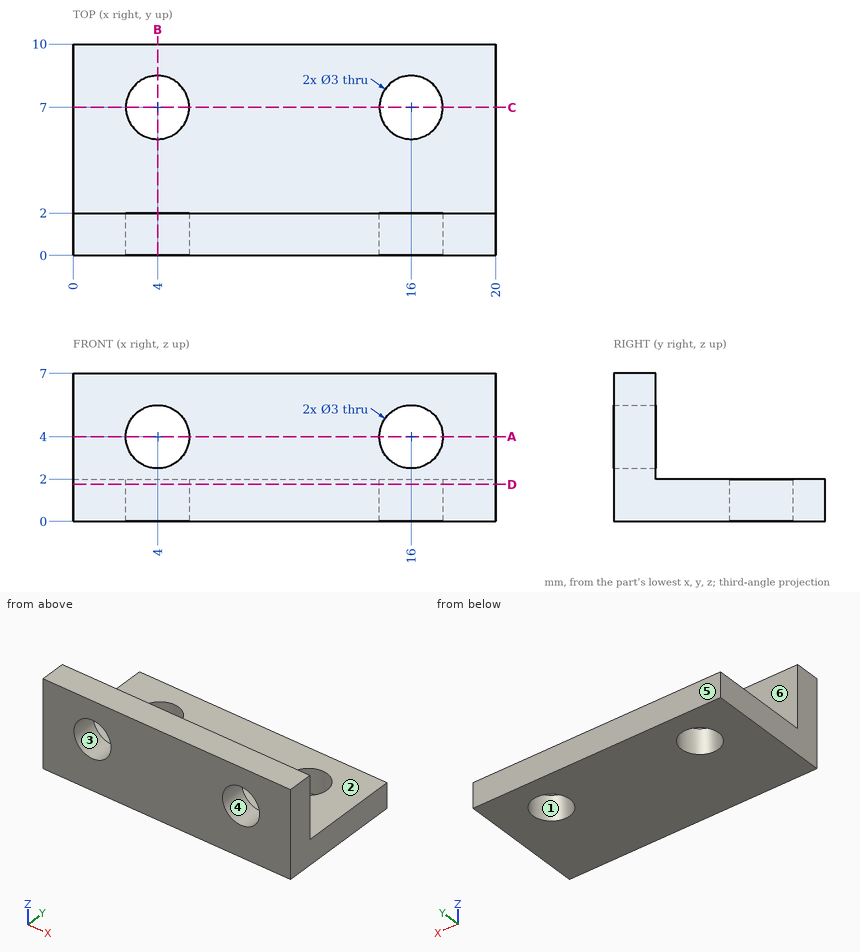
Part print with two shaded views. Sizes in mm from the minimum x, y, z corner. A direction names the side the tool comes from. Round coordinates to 2 decimals unless told otherwise and drop trailing zeros. Order: outer loops, then holes, each group sorted by start corner. A loop starts at its lowest first (then second) coordinate and runs counter-clockwise, first axis right, second up.
(1) Band-saw the part on B-B (x = 4). List the corners of the cut face in (y, z), then the cut area to 3 significant figures.
(2) Pin check, flat tips, straight feed: pin 1 (1 mm diameter, centred on x = 17.5, z = 5, fed in from +Y); pin 2 (4 mm diameter, centred on x = 9, y = 5, fed in from +Z). Stop position of each tip, or through.
(3) Band-saw the part on D-D (z = 1.75). List the corners of the cut face in (x, y).
(4) Drill centre lines: line 1 (Y direction, x = 4, z = 1); line 2 (X direction, y = 1, z = 4); line 3 (Z direction, x = 16, y = 1.4). Where is each one in solid material? Low to high.
(5) Pull direction Z, two halves, no side cores. Call the marked faces 1, 2, 3 and 4: released by +Z, released by -Z, zero draft, split by the parting line, or undercut.
(6) Band-saw the part on A-A (z = 4). List the corners of the cut face in (x, y), then the cut area to 3 significant figures.
(7) 3-axis set-ups, long thin cutter, end or side, ignore diameter. For the marked faces 5 and 6: which of +Z, -Z, +X, -X, +Y, -Y reach the whole face in a straight line?
Verdict:
1. outline: (0, 0) - (5.5, 0) - (5.5, 2) - (2, 2) - (2, 2.5) - (0, 2.5) - close; (0, 5.5) - (2, 5.5) - (2, 7) - (0, 7) - close; (8.5, 0) - (10, 0) - (10, 2) - (8.5, 2) - close
1. area: 18.0 mm2
2. pin 1: stops at y = 2
2. pin 2: stops at z = 2
3. outline: (0, 0) - (20, 0) - (20, 10) - (0, 10) - close; hole circle Ø3 at (4, 7); hole circle Ø3 at (16, 7)
4. line 1: y = 0 to 5.5, 8.5 to 10
4. line 2: x = 0 to 2.5, 5.5 to 14.5, 17.5 to 20
4. line 3: z = 0 to 2.5, 5.5 to 7
5. face 1: zero draft
5. face 2: released by +Z
5. face 3: undercut
5. face 4: undercut
6. outline: (0, 0) - (2.5, 0) - (2.5, 2) - (0, 2) - close; (5.5, 0) - (14.5, 0) - (14.5, 2) - (5.5, 2) - close; (17.5, 0) - (20, 0) - (20, 2) - (17.5, 2) - close
6. area: 28.0 mm2
7. face 5: +Z, -Z, +X, -X, +Y
7. face 6: +Z, +X, -X, +Y
